The listing builds one solid part. Answer for the finished solid, in the listing's coordinates (mm). A direction names the side the tool comes from. Coordinates: 2 decimals unless noted, no trailing zeros. Loops run counter-clockwise (first coordinate to the right, second up) from the corner with the lowest first, then second, coordinate; pieces in that order, holes last. Notation, with made-up numbers: M -11.75,51.25 L 44.25,51.25 A12 ccw 44.25,62.25 Z; hole C -22,-35 d8. An arc over 180 degrees is marked long. Answer in a Markdown table with one row per item. Add a question column.
from build123d import *

# Parameters (mm, degrees)
F1_DEPTH = 20
F3_DEPTH = 1


with BuildPart() as f1:
    # F0 (on Top) → F1 (new body)
    with BuildSketch(Plane.XY):
        with BuildLine():
            Line((0.5, 17), (-0.5, 17))
            Line((-0.5, 17), (-0.5, 2.598076))
            ThreePointArc((-0.5, 2.598076), (-1.035898, 0.598076), (-2.5, -0.866025))
            Line((-2.5, -0.866025), (-14.972432, -8.066987))
            Line((-14.972432, -8.066987), (-14.472432, -8.933013))
            Line((-14.472432, -8.933013), (-2, -1.732051))
            ThreePointArc((-2, -1.732051), (0, -1.196152), (2, -1.732051))
            Line((2, -1.732051), (14.472432, -8.933013))
            Line((14.472432, -8.933013), (14.972432, -8.066987))
            Line((14.972432, -8.066987), (2.5, -0.866025))
            ThreePointArc((2.5, -0.866025), (1.035898, 0.598076), (0.5, 2.598076))
            Line((0.5, 2.598076), (0.5, 17))
        make_face()
        with BuildLine():
            Line((1.5, 18), (-1.5, 18))
            Line((-1.5, 18), (-1.5, 2.598076))
            ThreePointArc((-1.5, 2.598076), (-1.901924, 1.098076), (-3, 0))
            Line((-3, 0), (-16.338457, -7.700962))
            Line((-16.338457, -7.700962), (-14.838457, -10.299038))
            Line((-14.838457, -10.299038), (-1.5, -2.598076))
            ThreePointArc((-1.5, -2.598076), (0, -2.196152), (1.5, -2.598076))
            Line((1.5, -2.598076), (14.838457, -10.299038))
            Line((14.838457, -10.299038), (16.338457, -7.700962))
            Line((16.338457, -7.700962), (3, 0))
            ThreePointArc((3, 0), (1.901924, 1.098076), (1.5, 2.598076))
            Line((1.5, 2.598076), (1.5, 18))
        make_face()
        with BuildLine():
            Line((-0.5, 2.598076), (-0.5, 17))
            Line((-0.5, 17), (0.5, 17))
            Line((0.5, 17), (0.5, 2.598076))
            ThreePointArc((0.5, 2.598076), (1.035898, 0.598076), (2.5, -0.866025))
            Line((2.5, -0.866025), (14.972432, -8.066987))
            Line((14.972432, -8.066987), (14.472432, -8.933013))
            Line((14.472432, -8.933013), (2, -1.732051))
            ThreePointArc((2, -1.732051), (0, -1.196152), (-2, -1.732051))
            Line((-2, -1.732051), (-14.472432, -8.933013))
            Line((-14.472432, -8.933013), (-14.972432, -8.066987))
            Line((-14.972432, -8.066987), (-2.5, -0.866025))
            ThreePointArc((-2.5, -0.866025), (-1.035898, 0.598076), (-0.5, 2.598076))
        make_face(mode=Mode.SUBTRACT)
    extrude(amount=F1_DEPTH)

    # F2 (on face) → F3 (join)
    with BuildSketch(Plane(origin=(0, 0, 0), x_dir=(1, 0, 0), z_dir=(0, 0, -1))):
        with BuildLine():
            Line((-0.5, -2.598076), (-0.5, -17))
            Line((-0.5, -17), (0.5, -17))
            Line((0.5, -17), (0.5, -2.598076))
            ThreePointArc((0.5, -2.598076), (1.035898, -0.598076), (2.5, 0.866025))
            Line((2.5, 0.866025), (14.972432, 8.066987))
            Line((14.972432, 8.066987), (14.472432, 8.933013))
            Line((14.472432, 8.933013), (2, 1.732051))
            ThreePointArc((2, 1.732051), (0, 1.196152), (-2, 1.732051))
            Line((-2, 1.732051), (-14.472432, 8.933013))
            Line((-14.472432, 8.933013), (-14.972432, 8.066987))
            Line((-14.972432, 8.066987), (-2.5, 0.866025))
            ThreePointArc((-2.5, 0.866025), (-1.035898, -0.598076), (-0.5, -2.598076))
        make_face()
    extrude(amount=-F3_DEPTH)


solid = f1.part
(1) A cutting plane is placed at C-C (y = 14). Give the vertices of the cut face in (x, z).
(2) Straight lines are drawn through the part: line 1 (X direction, y = 10.25, z = 17.25); line 2 (X direction, y = -5.5, z = 16.5); line 3 (Y direction, x = -10, z = 9.25). For each, find the intervals that lie inside material, in ascending order.
(3) A cutting plane is placed at A-A (z = 13). Give the vertices of the cut face in (x, y).
(4) A cutting plane is placed at B-B (y = -3). Give the vertices of the cut face in (x, z).
(5) The mould has two halves that part along X. Classify faces 5 (the face through (0, 1, 0)), 6 (the face through (8.32, -5.38, 10.37)), 7 (the face through (1.9, 1.1, 9.9)): released by +X, released by -X, zero draft, split by the parting line, or undercut.
(6) A cutting plane is placed at D-D (x = -7.5). Give the vertices of the cut face in (y, z), plus the area to 3 significant figures.
(7) For faces 1 (the face through (1.5, 10, 10)), 2 (the face through (-8.26, -6.5, 9.86)), 3 (the face through (0, 17, 10)), 4 (the face through (15.578, -9.018, 9.86)), determine the directions among +Z, -Z, +X, -X, +Y, -Y from which every point of the face is accessible in a straight line to the end or side of a thin tool.
(8) Each of these flat-tipped pins is pushed along its axis until it touches: pin 1 (0.5 mm diameter, centred on x = 0, z = 7.5, fed in from -Y); pin 2 (4 mm diameter, centred on x = 3, z = 17, fed in from -Y); pin 3 (1 mm diameter, centred on y = 8.5, z = 2.5, fed in from +X). Where does it stop, or does it pass through?
Solved:
| question | item | result |
|---|---|---|
| 1 | outline | M -1.5,0 L 1.5,0 L 1.5,20 L 0.5,20 L 0.5,1 L -0.5,1 L -0.5,20 L -1.5,20 Z |
| 2 | line 1 | x = -1.5 to -0.5, 0.5 to 1.5 |
| 2 | line 2 | x = -12.53 to -10.53, -8.53 to -6.53, 6.53 to 8.53, 10.53 to 12.53 |
| 2 | line 3 | y = -7.51 to -6.35, -5.2 to -4.04 |
| 3 | outline | M -16.34,-7.7 L -14.84,-10.3 L -1.5,-2.6 A3 cw 1.5,-2.6 L 14.84,-10.3 L 16.34,-7.7 L 3,0 A3 cw 1.5,2.6 L 1.5,18 L -1.5,18 L -1.5,2.6 A3 cw -3,0 Z; hole M -14.97,-8.07 L -14.47,-8.93 L -2,-1.73 A4 cw 2,-1.73 L 14.47,-8.93 L 14.97,-8.07 L 2.5,-0.87 A4 cw 0.5,2.6 L 0.5,17 L -0.5,17 L -0.5,2.6 A4 cw -2.5,-0.87 Z |
| 4 | outline | M -8.2,0 L -2.2,0 L -2.2,20 L -4.2,20 L -4.2,1 L -6.2,1 L -6.2,20 L -8.2,20 Z; M 2.2,0 L 8.2,0 L 8.2,20 L 6.2,20 L 6.2,1 L 4.2,1 L 4.2,20 L 2.2,20 Z |
| 5 | face 5 | zero draft |
| 5 | face 6 | undercut |
| 5 | face 7 | released by +X |
| 6 | outline | M -6.06,0 L -2.6,0 L -2.6,20 L -3.75,20 L -3.75,1 L -4.91,1 L -4.91,20 L -6.06,20 Z |
| 6 | area | 47.3 mm² |
| 7 | face 1 | +Z, -Z, +X, +Y |
| 7 | face 2 | +Z, -Z, -Y |
| 7 | face 3 | +Z |
| 7 | face 4 | +Z, -Z, +X, -Y |
| 8 | pin 1 | stops at y = -2.21 |
| 8 | pin 2 | stops at y = -4.62 |
| 8 | pin 3 | stops at x = 1.5 |
